Part model, mm, in its own coordinate system. Round coordinates to 2 decimals unless told otherwise and drop trailing zeros. Loops run counter-clockwise (first coordinate to the right, second up) from the corner with the lowest first, then second, coordinate; pieces in that order, holes last. Notation, with made-up numbers: (-13, 34) -> (34, 34) arc R12 ccw to (34, 49) -> close; hole circle Ø9 at (42, -10). An arc over 180 degrees is marked (long way). Answer as CSV lines item,"result".
Autodesk Fusion 360 part; units mm, degrees
sketch "Sketch1" plane through (0, 0, 0) normal (0, 0, 1) x (1, 0, 0)
  line L0 (0, 0) -> (127.5, 0)
  line L1 (127.5, 0) -> (127.5, 70)
  line L2 (127.5, 70) -> (0, 70)
  line L3 (0, 70) -> (0, 0)
  circle A0 centre (4, 35.763) radius 1.55
  line L4 (63.75, 0) -> (63.75, 70) construction
  circle A1 centre (123.5, 35.763) radius 1.55
  line L5 (66.25, 60) -> (61.25, 60)
  line L6 (61.25, 60) -> (61.25, 65)
  line L7 (61.25, 65) -> (66.25, 65)
  line L8 (66.25, 65) -> (66.25, 60)
  line L9 (66.25, 60) -> (61.25, 65) construction
  line L10 (61.25, 60) -> (66.25, 65) construction
  line L11 (63.75, 65) -> (61.25, 60)
  line L12 (63.75, 65) -> (66.25, 60)
  point P0 (63.75, 62.5)
  dimension "d1" = 127.5
  dimension "d2" = 70
  dimension "d3" = 3.1
  dimension "d4" = 35.763
  dimension "d5" = 4
  dimension "d8" = 5
  dimension "d9" = 5
  dimension "d12" = 5
extrude "Extrude1" add sketch "Sketch1" along normal blind 1.5 contours L0 L1 L2 L3 | L7 L8 L12 | L5 L11 L12 | L6 L7 L11
extrude "Extrude2" cut sketch "Sketch1" along normal blind 3 contours L5 L11 L12
sketch "Sketch2" plane through (0, 0, 1.5) normal (0, 0, 1) x (-1, 0, 0)
  line L0 (-63.75, -65) -> (-66.25, -60)
  line L1 (-66.25, -60) -> (-61.25, -60)
  line L2 (-61.25, -60) -> (-63.75, -65)
  circle A0 centre (-123.5, -35.763) radius 1.55
  circle A1 centre (-4, -35.763) radius 1.55
  line L3 (0, -70) -> (0, 0)
  line L4 (0, 0) -> (-127.5, 0)
  line L5 (-127.5, 0) -> (-127.5, -70)
  line L6 (-127.5, -70) -> (0, -70)
  line L7 (-90.5, -15) -> (-30.5, -15)
  line L8 (-30.5, -15) -> (-30.5, -55)
  line L9 (-30.5, -55) -> (-90.5, -55)
  line L10 (-90.5, -55) -> (-90.5, -15)
  line L11 (-90.5, -15) -> (-30.5, -55) construction
  line L12 (-30.5, -15) -> (-90.5, -55) construction
  circle A2 centre (-32.5, -53) radius 1.65
  circle A3 centre (-32.5, -53) radius 2.65
  circle A4 centre (-32.5, -17) radius 1.65
  circle A5 centre (-32.5, -17) radius 2.65
  circle A6 centre (-88.5, -53) radius 1.65
  circle A7 centre (-88.5, -53) radius 3.65
  circle A8 centre (-88.5, -17) radius 1.65
  circle A9 centre (-88.5, -17) radius 3.65
  line L13 (-123.5, -35.763) -> (-123.5, 0) construction
  line L14 (-123.5, -35.763) -> (-123.5, -70) construction
  line L15 (-125.5, -48) -> (-125.5, -60)
  arc A10 (-125.5, -60) -> (-121.5, -60) centre (-123.5, -60) ccw
  line L16 (-121.5, -60) -> (-121.5, -48)
  arc A11 (-121.5, -48) -> (-125.5, -48) centre (-123.5, -48) ccw
  line L17 (-123.5, -48) -> (-123.5, -60) construction
  point P0 (-60.5, -35)
  dimension "d13" = 40
  dimension "d14" = 60
  dimension "d15" = 15
  dimension "d16" = 37
  dimension "d17" = 3.3
  dimension "d18" = 5.3
  dimension "d19" = 2
  dimension "d20" = 2
  dimension "d21" = 3.3
  dimension "d22" = 5.3
  dimension "d23" = 2
  dimension "d24" = 2
  dimension "d25" = 3.3
  dimension "d26" = 7.3
  dimension "d27" = 2
  dimension "d28" = 2
  dimension "d29" = 3.3
  dimension "d30" = 7.3
  dimension "d31" = 2
  dimension "d32" = 2
  dimension "d37" = 4
  dimension "d38" = 10
  dimension "d39" = 12
extrude "Extrude3" add sketch "Sketch2" along normal blind 3 contours L7 L10 A9 | L7 L10 A9 | L7 A5 | L7 L8 A5 | L9 L10 A7 | L9 L10 A7 | L8 A5 | L8 A3 | L8 L9 A3 | L9 A3 picked at (-32.5411, -15.1182) picked at (-32.5411, -54.8818)
extrude "Extrude4" cut sketch "Sketch2" against normal blind 4 contours A2 | A4 | A6 | A8
extrude "Extrude5" cut sketch "Sketch2" against normal blind 4 contours L15 A10 L16 A11
equation "d1 = 134 mm - 6 mm - 0.5 mm"
equation "d4 = 0.763 mm + 35 mm"
equation "d5 = 7 mm - 3 mm"
equation "d18 = d17 + 2 mm"
equation "d21 = d17"
equation "d22 = d18"
equation "d23 = d20"
equation "d24 = d19"
equation "d25 = d17"
equation "d26 = d25 + 4 mm"
equation "d27 = d19"
equation "d28 = d20"
equation "d29 = d25"
equation "d30 = d26"
equation "d31 = d28"
equation "d32 = d27"
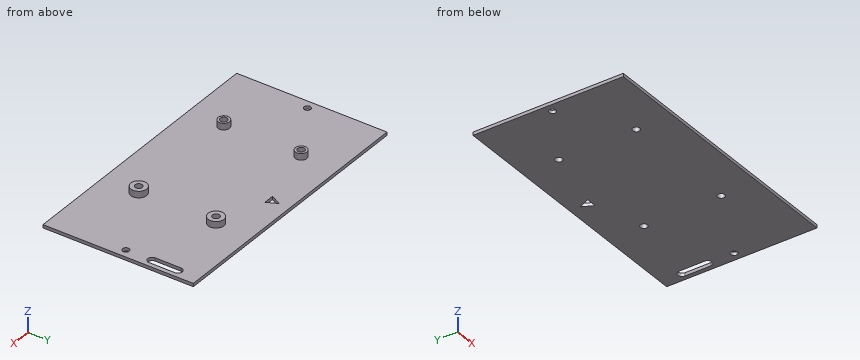
Q1. Saw through at D-D, the plane x = 4. Write the cut outline in (y, z), then the cut area to 3 significant figures.
Geometry results:
outline,"(0, 0) -> (34.21, 0) -> (34.21, 1.5) -> (0, 1.5) -> close; (37.31, 0) -> (70, 0) -> (70, 1.5) -> (37.31, 1.5) -> close"
area,"100 mm2"
Q2. Drill centre lines: line 1 along X through (y, z) = (53, 0.9); line 2 along Y through (x, z) = (32.5, 3.45); line 3 along X through (y, z) = (17, 1.2). Where is each one in solid material? Low to high.
Geometry results:
line 1,"0 to 30.85, 34.15 to 86.85, 90.15 to 121.5, 125.5 to 127.5"
line 2,"14.35 to 15.35, 18.65 to 19.65, 50.35 to 51.35, 54.65 to 55.65"
line 3,"0 to 30.85, 34.15 to 86.85, 90.15 to 127.5"
Q3. Saw through at A-A, the plane z = 2.55. Write the cut outline in (x, y).
Geometry results:
outline,"circle Ø5.3 at (32.5, 17); circle Ø5.3 at (32.5, 53); circle Ø7.3 at (88.5, 17); circle Ø7.3 at (88.5, 53); hole circle Ø3.3 at (32.5, 17); hole circle Ø3.3 at (32.5, 53); hole circle Ø3.3 at (88.5, 17); hole circle Ø3.3 at (88.5, 53)"
Q4. Saw through at C-C, the plane y = 53. Write the cut outline in (x, z).
Geometry results:
outline,"(0, 0) -> (30.85, 0) -> (30.85, 4.5) -> (29.85, 4.5) -> (29.85, 1.5) -> (0, 1.5) -> close; (34.15, 0) -> (86.85, 0) -> (86.85, 4.5) -> (84.85, 4.5) -> (84.85, 1.5) -> (35.15, 1.5) -> (35.15, 4.5) -> (34.15, 4.5) -> close; (90.15, 0) -> (121.5, 0) -> (121.5, 1.5) -> (92.15, 1.5) -> (92.15, 4.5) -> (90.15, 4.5) -> close; (125.5, 0) -> (127.5, 0) -> (127.5, 1.5) -> (125.5, 1.5) -> close"
Q5. Saw through at B-B, the plane x = 123.5. Write the cut outline in (y, z).
Geometry results:
outline,"(0, 0) -> (34.21, 0) -> (34.21, 1.5) -> (0, 1.5) -> close; (37.31, 0) -> (46, 0) -> (46, 1.5) -> (37.31, 1.5) -> close; (62, 0) -> (70, 0) -> (70, 1.5) -> (62, 1.5) -> close"
Q6. Drop a flat-ended pin along its axis: P1, Ø2, axis at x = 50.5, y = 59, coming from the +Z side. Give the stop position or say it passes through.
Geometry results:
P1,"z = 1.5"
